from build123d import *

# Parameters (mm, degrees)
SKETCH15_R         = 100
SKETCH15_R_2       = 81.5
BASE_FLANGE1_DEPTH = 1


# Read off the part's stored shape, not the designer's step: Edge-Flange1
# Sheet-metal steps are written as plain solids
with BuildPart() as part:
    # Sketch15 → Base-Flange1 (new body)
    with BuildSketch(Plane(origin=(0, 0, 0), x_dir=(1, 0, 0), z_dir=(0, 1, 0))):
        with Locations(Location((0, 0, 0), (0, 0, 270))):
            Circle(SKETCH15_R)
        with Locations(Location((0, 0, 0), (0, 0, 270))):
            Circle(SKETCH15_R_2, mode=Mode.SUBTRACT)
    extrude(amount=-BASE_FLANGE1_DEPTH)

    # Edge-Flange1 outline → Edge-Flange1 (revolve)
    with BuildSketch(Plane.XY):
        with BuildLine():
            Line((80.5, -1), (81.5, -1))
            Line((81.5, -1), (81.5, 0))
            Line((81.5, 0), (80.5, 0))
            ThreePointArc((80.5, 0), (78.378679656, 0.878679656), (77.5, 3))
            Line((77.5, 3), (77.5, 44))
            Line((77.5, 44), (76.5, 44))
            Line((76.5, 44), (76.5, 3))
            ThreePointArc((76.5, 3), (77.671572875, 0.171572875), (80.5, -1))
        make_face()
    revolve(axis=Axis((0, 0, 0), (0, 1, 0)))


solid = part.part
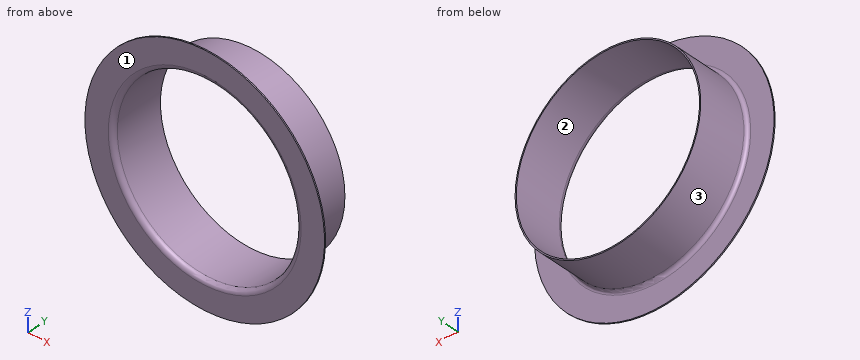
Input: part model. Units: mm. Frame: model coordinates. Face numbers are marked on the shaded views. Give positions to 0.01 mm unless a question says otherwise; leave off trailing zeros. Order: outer loops, then holes, each group sorted by start corner. A loop starts at its lowest first (then second) coordinate and runs counter-clockwise, first axis right, second up. Notation, with made-up numbers: (-4.75, 43.5) - (50.25, 43.5) arc R22 cw to (50.25, 51.5) - close; hole circle Ø8 at (4.5, 88). An arc over 180 degrees is marked (long way). Answer as a JSON object with one key per item and string values. Group by question number.
Q1. First-contact query: pin 1 Ø12 at (x, y) = (10, 25) entering from -Z; pin 2 Ø1 at (y, z) = (30, -66.5) entering from -X; pin 3 Ø3 at (x, y) = (32, 13) entering from +Z. Flat tips, straight axial feed; report the tip coordinate or a pass-through.
Q2. Cut plane B-B, the plane z = 0. Output: boundary loops of the cut face in (x, y).
Q3. Cut plane C-C, the plane y = 14.5. Output: boundary loops of the cut face in (x, z).
Q4. Mould query, pull axis Z, two halves, no side actions, for the marked faces 1, 2 and 3. Classes: pulls with the +Z half, pulls with the -Z half, needs draft (parallel to the pull), parting line crosses it, or undercut.
Q5. Line query: probe 1 along X at (y, z) = (19, 0); probe 2 along Y at (x, z) = (-71, 39). Output: solid intervals per line, ascending.
Q6. Cut plane A-A, the plane x = 0. Output: boundary loops of the cut face in (y, z).
Results:
{
 "1": {"pin 1": "z = -77.4", "pin 2": "x = -40.62", "pin 3": "z = 71.25"},
 "2": {"outline": "(-100, -1) - (-80.5, -1) arc R4 ccw to (-76.5, 3) - (-76.5, 44) - (-77.5, 44) - (-77.5, 3) arc R3 cw to (-80.5, 0) - (-100, 0) - close; (76.5, 3) arc R4 ccw to (80.5, -1) - (100, -1) - (100, 0) - (80.5, 0) arc R3 cw to (77.5, 3) - (77.5, 44) - (76.5, 44) - close"},
 "3": {"outline": "circle Ø155 at (0, 0); hole circle Ø153 at (0, 0)"},
 "4": {"face 1": "needs draft", "face 2": "undercut", "face 3": "parting line crosses it"},
 "5": {"probe 1": "-77.5 to -76.5, 76.5 to 77.5", "probe 2": "-1 to 0"},
 "6": {"outline": "(-1, -100) - (0, -100) - (0, -80.5) arc R3 cw to (3, -77.5) - (44, -77.5) - (44, -76.5) - (3, -76.5) arc R4 ccw to (-1, -80.5) - close; (-1, 80.5) arc R4 ccw to (3, 76.5) - (44, 76.5) - (44, 77.5) - (3, 77.5) arc R3 cw to (0, 80.5) - (0, 100) - (-1, 100) - close"}
}
